Geometry: final body of the model. Coordinates: model frame, mm. Face numbers are marked on the shaded views. A direction names the side the tool comes from. Give positions to 0.01 mm unless a question says otherwise; leave off trailing zeros. Write each loop counter-clockwise with the first axis right and the second up, starting at its lowest first coordinate (ties: lowest second). Pieces come first, ordered by that corner, then holes. Notation, with made-up numbers: (-13, 67.5) - (15, 67.5) arc R35 cw to (15, 104.5) - close; hole circle Ø11 at (-26, -36.75). An arc over 180 degrees is marked (long way). One line per question, with ' | ' between items. Start each with the question number.
```python
from build123d import *

# Parameters (mm, degrees)
SKETCH1_W           = 11.3
SKETCH1_H           = 3
SKETCH1_W_2         = 3
SKETCH1_H_2         = 12.5
BOSS_EXTRUDE1_DEPTH = 9
FILLET1_R           = 1.5
SKETCH2_W           = 7.5
SKETCH2_H           = 3
BOSS_EXTRUDE2_DEPTH = 12


with BuildPart() as part:
    # Sketch1 → Boss-Extrude1 (new body)
    with BuildSketch(Plane(origin=(0, 0, 0), x_dir=(1, 0, 0), z_dir=(0, 1, 0))):
        Polygon((-8.65, -1.5), (-5.65, -1.5), (-5.65, 1.5), (-5.65, 18.5), (-8.65, 18.5), align=None)
        Rectangle(SKETCH1_W, SKETCH1_H)
        Polygon((3.65, 1.5), (5.65, 1.5), (5.65, 6), (3.65, 6), (3.65, 3), align=None)
        Polygon((-4.15, 3), (3.65, 3), (3.65, 6), (-1.15, 6), (-4.15, 6), align=None)
        with Locations((-2.65, 12.25)):
            Rectangle(SKETCH1_W_2, SKETCH1_H_2)
    extrude(amount=BOSS_EXTRUDE1_DEPTH)

    # Fillet1
    fillet1_edges = [part.edges().sort_by_distance(p)[0] for p in [
        (-4.15, 4.5, -3),
    ]]
    fillet(fillet1_edges, radius=FILLET1_R)

    # Sketch2 → Boss-Extrude2 (add)
    with BuildSketch(Plane(origin=(5.65, 0, 0), x_dir=(0, 0, -1), z_dir=(1, 0, 0))):
        with Locations((2.25, 4.5)):
            Rectangle(SKETCH2_W, SKETCH2_H)
    extrude(amount=BOSS_EXTRUDE2_DEPTH)


solid = part.part
```
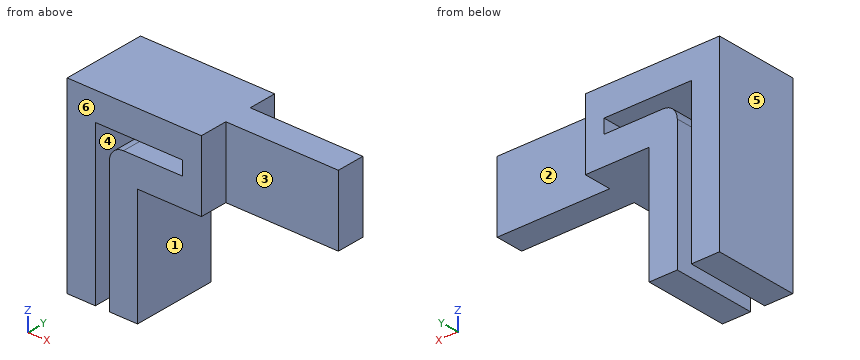
1) Pull-direction query (X, two-part tool) for the marked faces 4, 5 and 6; classes: +X half, -X half, draft (parallel to the pull), parting line (faces both ways), or undercut.
2) Section B-B, the plane x = 2. Output: boundary loops of the cut face in (y, z).
3) Section A-A, the plane z = -10.75. Output: boundary loops of the cut face in (x, y), plus the area to 3 significant figures.
4) First-contact query: pin 1 Ø6 at (x, z) = (10, -1.5) entering from +Y; pin 2 Ø4 at (x, y) = (14, 3.5) entering from -Z; pin 3 Ø2.5 at (y, z) = (1, -4) entering from +X. Flat tips, straight axial feed; report the tip coordinate or a pass-through.
5) Reachability of the marked faces 1, 2 and 3 from +Z, -Z, +X, -X, +Y, -Y: full face, straight path, thin tool, end or side. Return the list, or none.
6) Line query: L1, parallel to Z at x = 2.5, y = 5.5; L2, parallel to X at y = 3, z = -15.5; L3, parallel to X at y = 5, z = -4.5. Output: solid intervals per line, ascending.
7) Section C-C, the plane y = 6.75. Output: boundary loops of the cut face in (x, z), plus the area to 3 significant figures.
8) Section D-D, the plane x = 15. Output: boundary loops of the cut face in (y, z), plus the area to 3 significant figures.
Answer key:
1) face 4: undercut | face 5: -X half | face 6: draft
2) outline: (0, -6) - (9, -6) - (9, -3) - (0, -3) - close; (0, -1.5) - (9, -1.5) - (9, 1.5) - (0, 1.5) - close
3) outline: (-8.65, 0) - (-5.65, 0) - (-5.65, 9) - (-8.65, 9) - close; (-4.15, 0) - (-1.15, 0) - (-1.15, 9) - (-4.15, 9) - close | area: 54.0 mm^2
4) pin 1: y = 6 | pin 2: z = -6 | pin 3: x = 5.65
5) face 1: -Z, +X, +Y, -Y | face 2: +Z, -Z, +X, +Y | face 3: +Z, -Z, +X, -Y
6) L1: -6 to -3, -1.5 to 1.5 | L2: -8.65 to -5.65, -4.15 to -1.15 | L3: -8.65 to -5.65, -4.15 to 17.65
7) outline: (-8.65, -18.5) - (-5.65, -18.5) - (-5.65, -1.5) - (3.65, -1.5) - (3.65, -3) - (-2.65, -3) arc R1.5 ccw to (-4.15, -4.5) - (-4.15, -18.5) - (-1.15, -18.5) - (-1.15, -6) - (5.65, -6) - (5.65, 1.5) - (-8.65, 1.5) - close | area: 163 mm^2
8) outline: (3, -6) - (6, -6) - (6, 1.5) - (3, 1.5) - close | area: 22.5 mm^2
